from build123d import *

# Parameters (mm, degrees)
F1_DEPTH  = 1.5
F3_DEPTH  = 25
F4_DEPTH  = 5
F6_W      = 90
F6_H      = 3
F7_DEPTH  = 5
F5_R      = 1.75
F8_DEPTH  = 3.8
F9_W      = 16.7752551286
F9_H      = 3
F9_W_2    = 2.4494897428
F9_W_3    = 49.5505102572
F9_W_4    = 18.7752551286
F10_DEPTH = 10
F15_DEPTH = 5.301


# Not quite as in the source:
# - ends of sketch curves that miss each other by under 0.0002 mm in the source are joined


with BuildPart() as f1:
    # F0 (on Front) → F1 (new body)
    with BuildSketch(Plane.XZ):
        Polygon((0, -0.8), (0, -1.5), (3, -1.2631578947), (2.9450791466, -0.5674937516), align=None)
        Polygon((2.9450791466, -0.5674937516), (3, -1.2631578947), (19, 0), (10.1333333333, 0), (8, -0.1684210526), align=None)
        Polygon((0, 0), (0, -0.8), (2.9450791466, -0.5674937516), (8, -0.1684210526), (7.9867036011, 0), align=None)
        Polygon((10.1333333333, 0), (19, 0), (3, 1.2631578947), (2.9450791466, 0.5674937516), (8, 0.1684210526), align=None)
        Polygon((0, 0.8), (0, 0), (7.9867036011, 0), (8, 0.1684210526), (2.9450791466, 0.5674937516), align=None)
        Polygon((2.9450791466, 0.5674937516), (3, 1.2631578947), (0, 1.5), (0, 0.8), align=None)
        Polygon((8, -0.1684210526), (10.1333333333, 0), (7.9867036011, 0), align=None)
        Polygon((7.9867036011, 0), (10.1333333333, 0), (8, 0.1684210526), align=None)
    extrude(amount=-F1_DEPTH)

    # F2 (on face) → F3 (cut)
    with BuildSketch(Plane(origin=(0.117687543, 0, 1.4907088782), x_dir=(0.9968981487, 0, -0.0787024854), z_dir=(0.0787024854, 0, 0.9968981487))):
        Polygon((18.9410648244, 1.5), (-0.1180537281, 1.5), (18.9410648244, 0), align=None)
    extrude(amount=-F3_DEPTH, mode=Mode.SUBTRACT)

    # F0 (on Front) → F4 (join)
    with BuildSketch(Plane.XZ):
        Polygon((0, 0.8), (0, 0), (7.9867036011, 0), (8, 0.1684210526), (2.9450791466, 0.5674937516), align=None)
        Polygon((0, 0), (0, -0.8), (2.9450791466, -0.5674937516), (8, -0.1684210526), (7.9867036011, 0), align=None)
        Polygon((0, -0.8), (0, -1.5), (3, -1.2631578947), (2.9450791466, -0.5674937516), align=None)
        Polygon((2.9450791466, 0.5674937516), (3, 1.2631578947), (0, 1.5), (0, 0.8), align=None)
    extrude(amount=-F4_DEPTH)

    # F6 (on face) → F7 (join, through all)
    with BuildSketch(Plane.XZ):
        with Locations((-45, 0)):
            Rectangle(F6_W, F6_H)
    extrude(amount=-F7_DEPTH)

    # F5 (on Top) → F8 (join, symmetric)
    with BuildSketch(Plane.XY):
        with Locations((-20, 6.25)):
            Circle(F5_R)
        with Locations((-72, 6.25)):
            Circle(F5_R)
    extrude(amount=F8_DEPTH, both=True)

    # F9 (on face) → F10 (join)
    with BuildSketch(Plane(origin=(0, 5, 0), x_dir=(-1, 0, 0), z_dir=(0, 1, 0))):
        with Locations((81.6123724357, 0)):
            Rectangle(F9_W, F9_H)
        with Locations((72, 0)):
            Rectangle(F9_W_2, F9_H)
        with Locations((46, 0)):
            Rectangle(F9_W_3, F9_H)
        with Locations((20, 0)):
            Rectangle(F9_W_2, F9_H)
        with Locations((9.3876275643, 0)):
            Rectangle(F9_W_4, F9_H)
    extrude(amount=F10_DEPTH)

    # F13: sweep along a path in F11
    with BuildLine(Plane.XY) as f13_path:
        Line((-90, 2), (6, 0))
    # F12 (on face) → F13 (sweep, cut)
    with BuildSketch(Plane(origin=(-90, 0, 0), x_dir=(0, -1, 0), z_dir=(-1, 0, 0))):
        Polygon((-2, 0), (0, -1.5), (0, 1.5), align=None)
    sweep(path=f13_path.line, mode=Mode.SUBTRACT)

    # F14 (on face) → F15 (cut, through all)
    with BuildSketch(Plane.XY.offset(1.5)):
        Polygon((-90, 0.7), (-90, 0), (-10.954622702, 0), (-31, 0.7), align=None)
    extrude(amount=-F15_DEPTH, mode=Mode.SUBTRACT)


solid = f1.part
CAD build for the part. Positions are in the model's coordinates, mm. A direction names the side the tool comes from. Round coordinates to 2 decimals unless told otherwise and drop trailing zeros. Order: outer loops, then holes, each group sorted by start corner. A loop starts at its lowest first (then second) coordinate and runs counter-clockwise, first axis right, second up. Notation, with made-up numbers: (78, -18.75) - (107, -18.75) arc R17 cw to (107, -2.75) - close; hole circle Ø1 at (17, -26.75). An arc over 180 degrees is marked (long way). Return JSON: item names as keys, results as strings.
(1) Cut at C-C (x = -37). Give the cut face in (y, z).
Answer key:
{"outline": "(0.7, -1.5) - (15, -1.5) - (15, 1.5) - (0.7, 1.5) - (0.7, 0.15) - (0.9, 0) - (0.7, -0.15) - close"}
(2) Cut at A-A (y = 6.25). Give the cut face in (x, z), then the cut area to 3 significant figures.
Answer key:
{"outline": "(-90, -1.5) - (-73.75, -1.5) - (-73.75, -3.8) - (-70.25, -3.8) - (-70.25, -1.5) - (-21.75, -1.5) - (-21.75, -3.8) - (-18.25, -3.8) - (-18.25, -1.5) - (0, -1.5) - (0, 1.5) - (-18.25, 1.5) - (-18.25, 3.8) - (-21.75, 3.8) - (-21.75, 1.5) - (-70.25, 1.5) - (-70.25, 3.8) - (-73.75, 3.8) - (-73.75, 1.5) - (-90, 1.5) - close", "area": "302 mm^2"}
(3) Tool access for faces 1 (the face through (0, 10, 0)), 2 (the face through (-21.4, 5.2, -2.6)), 3 (the face through (-21.4, 5.2, 2.6)): list every direction of +Z, -Z, +X, -X, +Y, -Y with a clear straight run to the whole face (end or side of a thin tool).
Answer key:
{"face 1": "+Z, -Z, +X, +Y", "face 2": "-Z", "face 3": "+Z"}
(4) Pin check, flat tips, straight feed: pin 1 Ø1.2 at (x, z) = (-63, 0.5) entering from -Y; pin 2 Ø2.5 at (x, z) = (4, 0) entering from +Y; pin 3 Ø2.5 at (y, z) = (10.5, 0) entering from +X. Stop position of each tip, or through.
Answer key:
{"pin 1": "stops at y = 0.7", "pin 2": "stops at y = 5", "pin 3": "stops at x = 0"}
(5) Wall check: probe 1 along Z at (x, y) = (-11, 7.5); probe 2 along X at (y, z) = (6.5, -3); probe 3 along X at (y, z) = (14.25, 1.25). Give the ranges that are in metal, low to high. Write a range as from..to.
Answer key:
{"probe 1": "z = -1.5..1.5", "probe 2": "x = -73.73..-70.27, -21.73..-18.27", "probe 3": "x = -90..0"}
(6) Cut at D-D (x = -79). Give the cut face in (y, z).
Answer key:
{"outline": "(0.7, -1.5) - (15, -1.5) - (15, 1.5) - (0.7, 1.5) - (0.7, 0.8) - (1.77, 0) - (0.7, -0.8) - close"}
(7) Cut at B-B (z = -2.75). Give the cut face in (x, y).
Answer key:
{"outline": "circle Ø3.5 at (-72, 6.25); circle Ø3.5 at (-20, 6.25)"}
